Part model, mm, in its own coordinate system. A direction names the side the tool comes from. Coordinates: 2 decimals unless noted, no trailing zeros. Loops run counter-clockwise (first coordinate to the right, second up) from the corner with the lowest first, then second, coordinate; pieces in that order, holes last.
```python
from build123d import *

# Parameters (mm, degrees)
SKETCH1_R               = 45
SKETCH1_R_2             = 35
BOSS_EXTRUDE1_DEPTH     = 37.21
FILLET1_R               = 10
SKETCH3_W               = 3.623403209
SKETCH3_H               = 6.465591727
CUT_EXTRUDE3_DEPTH      = 74.719632638
CUT_EXTRUDE3_DEPTH_BACK = 10
SKETCH4_R               = 1.161936473
SKETCH5_R               = 1.222255242
CUT_EXTRUDE4_DEPTH      = 10


with BuildPart() as part:
    # Sketch1 → Boss-Extrude1 (new body)
    with BuildSketch(Plane(origin=(0, 0, 0), x_dir=(1, 0, 0), z_dir=(0, 1, 0))):
        with Locations(Location((0, 0, 0), (0, 0, 270))):
            Circle(SKETCH1_R)
        with Locations(Location((0, 0, 0), (0, 0, 270))):
            Circle(SKETCH1_R_2, mode=Mode.SUBTRACT)
    extrude(amount=BOSS_EXTRUDE1_DEPTH)

    # Sketch2 → Cut-Revolve2 (revolve, cut)
    with BuildSketch(Plane(origin=(0, 0, 0), x_dir=(0, 0, -1), z_dir=(1, 0, 0)), mode=Mode.PRIVATE) as cut_revolve2_sk:
        Polygon((45, 18.605), (39.004948157, 0), (45, 0), align=None)
    revolve(cut_revolve2_sk.sketch.rotate(Axis((0, 37.21, 0), (0, -1, 0)), 180), axis=Axis((0, 37.21, 0), (0, -1, 0)), mode=Mode.SUBTRACT)

    # Fillet1
    fillet1_edges = [part.edges().sort_by_distance(p)[0] for p in [
        (0, 18.605, -45),
    ]]
    fillet(fillet1_edges, radius=FILLET1_R)

    # Sketch3 → Cut-Revolve3 (revolve, cut)
    with BuildSketch(Plane(origin=(0, 0, 0), x_dir=(0, 0, -1), z_dir=(1, 0, 0))):
        with Locations((-36.811701605, 9.799884952)):
            Rectangle(SKETCH3_W, SKETCH3_H)
    revolve(axis=Axis((0, 37.21, 0), (0, -1, 0)), mode=Mode.SUBTRACT)

    # Sketch4 → Cut-Extrude3 (cut, two sides: drawn at the far end of the back side and taken through both)
    with BuildSketch(Plane(origin=(0, 0, 0), x_dir=(-1, 0, 0), z_dir=(0, -1, 0)).offset(-CUT_EXTRUDE3_DEPTH_BACK)):
        with Locations(Location((36.80548689, 0, 0), (0, 0, 270))):
            Circle(SKETCH4_R)
    extrude(amount=CUT_EXTRUDE3_DEPTH + CUT_EXTRUDE3_DEPTH_BACK, mode=Mode.SUBTRACT)

    # Sketch5 → Cut-Extrude4 (cut)
    with BuildSketch(Plane(origin=(0, 0, 0), x_dir=(-1, 0, 0), z_dir=(0, -1, 0))):
        with Locations(Location((-36.771801863, 0, 0), (0, 0, 90))):
            Circle(SKETCH5_R)
    extrude(amount=-CUT_EXTRUDE4_DEPTH, mode=Mode.SUBTRACT)


solid = part.part
```
Q1. Mould opens along Y. For faces 1 (the flat face through (15, 0, -32)), 2 (the cylindrical face through (-11.6, 9.85, 36.84)), 3 (the cylindrical face through (-21, 3, -28)), 4 (the flat face through (-26.5, 37.21, 23.1)) say: released by +Y, released by -Y, zero draft, split by the parting line, or undercut.
Q2. Saw through at B-B (y = 32.5). List the corners of the cut face in (x, z), plus the area to 3 significant figures.
Q3. Tool access for faces 5 (the cylindrical face through (-37.958, 3.33, -0.151)), 6 (the flat face through (-6, 13.033, -35)), 7 (the cylindrical face through (-43.93, 28.57, -9.76)): list every direction of +Z, -Z, +X, -X, +Y, -Y with a clear straight run to the whole face (end or side of a thin tool).
Q4. Probe line 1 (Y direction, x = -15, z = 33); line 2 (X direction, y = 3, z = 0); line 3 (X direction, y = 27.5, z = 0). List the from-to ranges inside material, lowest first.
Q5. Saw through at C-C (y = 5). List the corners of the cut face in (x, z).
Q6. Saw through at A-A (z = 0). Count the separate pieces of the cut face and the enclosed holes in it, plus the area to 3 significant figures.
Q7. Drop flat-ended pins along their axis: P1, Ø1.5, axis at x = 26, y = 19, coming from the +Z side; P2, Ø12, axis at y = 24, z = -16.5, coming from the +X side; P3, Ø3, axis at x = 36.77, z = 0, coming from the -Y side; P4, Ø1.4, axis at x = -36.81, z = 0, coming from the -Y side. Give the stop position or say it passes through.
Q8. Saw through at D-D (y = 16). List the corners of the cut face in (x, z).
Checked values:
1. face 1: released by -Y
1. face 2: undercut
1. face 3: zero draft
1. face 4: released by +Y
2. outline: circle Ø90 at (0, 0); hole circle Ø70 at (0, 0)
2. area: 2,510 mm2
3. face 5: -Y
3. face 6: none
3. face 7: +Y, -Y
4. line 1: y = 0 to 6.57, 13.03 to 37.21
4. line 2: x = -39.97 to -37.97, -35.64 to -35, 35 to 35.55, 37.99 to 39.97
4. line 3: x = -45 to -35, 35 to 45
5. outline: circle Ø81.23 at (0, 0); hole circle Ø2.32 at (-36.81, 0); hole circle Ø70 at (0, 0); hole circle Ø2.44 at (36.77, 0)
6. separate pieces: 4
6. enclosed holes: 0
6. area: 554 mm2
7. P1: stops at z = 37.17
7. P2: stops at x = 43.76
7. P3: stops at y = 0
7. P4: stops at y = 13.03
8. outline: circle Ø88.32 at (0, 0); hole circle Ø70 at (0, 0)
